For this review, take the finished solid that the model builds, in its own axes (mm). Face numbers are marked on the shaded views. Coordinates: 2 decimals unless noted, no trailing zeros. Loops run counter-clockwise (first coordinate to the right, second up) from the corner with the lowest first, then second, coordinate; pieces in that order, holes last. Notation, with made-up numbers: M 77.5,-0.5 L 113.5,-0.5 A18 ccw 113.5,14.5 Z; hole C 51.25,-20.5 d3. An arc over 180 degrees is marked long. Use one line per item in the form item = value.
Autodesk Inventor part; units mm, degrees
ref_plane "Work Plane1" through (9, 0, 0) normal (1, 0, 0) x (0, 0, -1)
ref_plane "YZ Plane" through (0, 0, 0) normal (1, 0, 0) x (0, 1, 0)
ref_plane "XZ Plane" through (0, 0, 0) normal (0, 1, 0) x (-1, 0, 0)
sketch "Sketch1" plane through (0, 0, 0) normal (1, 0, 0) x (0, 1, 0)
  line L0 (-15, 75) -> (15, 75)
  line L1 (15, 75) -> (15, -75)
  line L2 (15, -75) -> (-15, -75)
  line L3 (-15, -75) -> (-15, 75)
  line L4 (-15, 75) -> (15, -75) construction
  line L5 (15, 75) -> (-15, -75) construction
  line L6 (15, 64.89637) -> (15, 43.985813)
  line L7 (-15, 43.985813) -> (-15, 64.193072)
  line L8 (-21, 0) -> (21, 0)
  line L9 (0, -105) -> (0, 105)
  line L10 (-15, -62.009619) -> (-7.5, -49.019238)
  line L11 (-7.5, -49.019238) -> (7.5, -49.019238)
  line L12 (7.5, -49.019238) -> (15, -62.009619)
  line L13 (15, -62.009619) -> (7.5, -75)
  line L14 (7.5, -75) -> (-7.5, -75)
  line L15 (-7.5, -75) -> (-15, -62.009619)
  line L16 (15, 62.009619) -> (7.5, 75)
  line L17 (-7.5, 75) -> (-15, 62.009619)
  point P0 (0, 0)
  point P1 (0, -62.009619)
  point P2 (-7.5, -75)
  point P3 (7.5, -75)
  point P4 (15, -62.009619)
  point P5 (15, 62.009619)
  point P6 (7.5, 75)
  point P7 (-7.5, 75)
  point P8 (-15, 62.009619)
  dimension "d0" = 30
  dimension "d1" = 150
extrude "Extrusion1" add sketch "Sketch1" along normal blind 4 contours L0 L9 L8 L3 L17 | L0 L16 L1 L8 L9 | L9 L11 L10 L3 L8 | L8 L1 L12 L11 L9 | L11 L12 L13 L2 L9 | L9 L2 L15 L10 L11
sketch "Sketch2" plane through (4, 0, 0) normal (1, 0, 0) x (0, 0, -1)
  line L0 (62.009619, 15) -> (-62.009619, 15)
  line L1 (62.009619, 15) -> (-62.009619, 15)
  line L2 (-62.009619, -15) -> (62.009619, -15)
  line L3 (-105, 0) -> (105, 0)
  line L4 (0, -21) -> (0, 21)
  line L5 (-68.504809, 4.618802) -> (-64.504809, 2.309401)
  line L6 (-64.504809, 2.309401) -> (-64.504809, -2.309401)
  line L7 (-64.504809, -2.309401) -> (-68.504809, -4.618802)
  line L8 (-68.504809, -4.618802) -> (-72.504809, -2.309401)
  line L9 (-72.504809, -2.309401) -> (-72.504809, 2.309401)
  line L10 (-72.504809, 2.309401) -> (-68.504809, 4.618802)
  line L11 (68.504809, 4.618802) -> (64.504809, 2.309401)
  line L12 (64.504809, 2.309401) -> (64.504809, -2.309401)
  line L13 (64.504809, -2.309401) -> (68.504809, -4.618802)
  line L14 (68.504809, -4.618802) -> (72.504809, -2.309401)
  line L15 (72.504809, -2.309401) -> (72.504809, 2.309401)
  line L16 (72.504809, 2.309401) -> (68.504809, 4.618802)
  line L17 (-75, 7.5) -> (-75, -7.5)
  line L18 (-62.009619, -15) -> (62.009619, -15)
  line L19 (-62.009619, 15) -> (-62.009619, -15)
  line L20 (-75, 7.5) -> (-75, -7.5)
  line L21 (-75, 0) -> (-62.009619, 0)
  point P0 (0, 0)
  point P1 (68.504809, 0)
  point P2 (-68.504809, 0)
  dimension "d8" = 8
sketch "Sketch2 outline for Extrusion3" plane through (4, 0, 0) normal (1, 0, 0) x (0, 0, -1)
  line L0 (68.504809, -4.618802) -> (72.504809, -2.309401)
  line L1 (64.504809, -2.309401) -> (68.504809, -4.618802)
  line L2 (64.504809, 2.309401) -> (64.504809, -2.309401)
  line L3 (68.504809, 4.618802) -> (64.504809, 2.309401)
  line L4 (72.504809, 2.309401) -> (68.504809, 4.618802)
  line L5 (72.504809, -2.309401) -> (72.504809, 2.309401)
  line L6 (-64.504809, 2.309401) -> (-68.504809, 4.618802)
  line L7 (-64.504809, -2.309401) -> (-64.504809, 2.309401)
  line L8 (-68.504809, -4.618802) -> (-64.504809, -2.309401)
  line L9 (-72.504809, -2.309401) -> (-68.504809, -4.618802)
  line L10 (-72.504809, 2.309401) -> (-72.504809, -2.309401)
  line L11 (-68.504809, 4.618802) -> (-72.504809, 2.309401)
extrude "Extrusion3" add sketch "Sketch2 outline for Extrusion3" along normal blind 15
sketch "Sketch3" plane through (19, 0, 0) normal (1, 0, 0) x (0, 0, -1)
  line L0 (-64.504809, 2.309401) -> (-68.504809, 4.618802)
  line L1 (-68.504809, -4.618802) -> (-64.504809, -2.309401)
  line L2 (-64.504809, -2.309401) -> (-64.504809, 2.309401)
  line L3 (-64.504809, -2.309401) -> (-68.504809, -4.618802)
  circle A0 centre (-68.504809, 0) radius 1.55
  line L4 (0, -21) -> (0, 21)
  circle A1 centre (68.504809, 0) radius 1.55
  line L5 (-68.504809, 4.618802) -> (-68.504809, -4.618802)
  point P0 (0, 0)
  dimension "d12" = 3.1
extrude "Extrusion4" cut sketch "Sketch3" against normal through all contours L5 A0 | A0 L5 | A1
ref_plane "Work Plane1" through (9, 0, 0) normal (1, 0, 0) x (0, 0, -1)
sketch "Sketch4" plane through (9, 0, 0) normal (-1, 0, 0) x (0, 0, 1)
  circle A0 centre (-68.504809, 0) radius 1.55
  circle A1 centre (68.504809, 0) radius 1.55
  circle A2 centre (-68.504809, 0) radius 3.05
  circle A3 centre (68.504809, 0) radius 3.05
  point P0 (0, 0)
  dimension "d15" = 6.1
sketch "Sketch4 outline for Extrusion5" plane through (9, 0, 0) normal (-1, 0, 0) x (0, 0, 1)
  circle A0 centre (68.504809, 0) radius 3.05
  circle A1 centre (-68.504809, 0) radius 3.05
extrude "Extrusion5" cut sketch "Sketch4 outline for Extrusion5" against normal blind 2.2 draft -32.5
sketch "Sketch5" plane through (0, 0, 0) normal (-1, 0, 0) x (0, 0, 1)
  circle A0 centre (-68.504809, 0) radius 3.05
  circle A1 centre (68.504809, 0) radius 3.05
  point P0 (0, 0)
extrude "Extrusion6" cut sketch "Sketch5" against normal up to surface (9 mm away)
sketch "Sketch8" plane through (0, 0, 0) normal (-1, 0, 0) x (0, 0, 1)
  circle A0 centre (-35, 0) radius 2.1
  line L0 (-75, -7.5) -> (-75, 7.5)
  line L1 (0, -21) -> (0, 21)
  line L2 (75, 7.5) -> (75, -7.5)
  line L3 (-105, 0) -> (105, 0)
  point P0 (0, 0)
  dimension "d26" = 40
  dimension "d27" = 4.2
extrude "Extrusion7" cut sketch "Sketch8" against normal through all
equation "\"d0\" = BodyHeight"
equation "\"d1\" = BodyLength"
equation "\"d2\" = SideThickness"
equation "\"d8\" = M3ScrewInsertBrim"
equation "\"d9\" = WheeGuardlSlotWidth"
equation "\"d12\" = M3ScrewDia"
equation "\"d15\" = M3ScrewHeadDia"
equation "\"d16\" = M3ScrewHeadDepth"
equation "\"d17\" = M3ScrewHeadTaper"
equation "\"d26\" = DriveMotorOffset"
equation "\"d27\" = DriveMotorHoleDia"
properties part number "HexWheelGuard" material "H TPU"
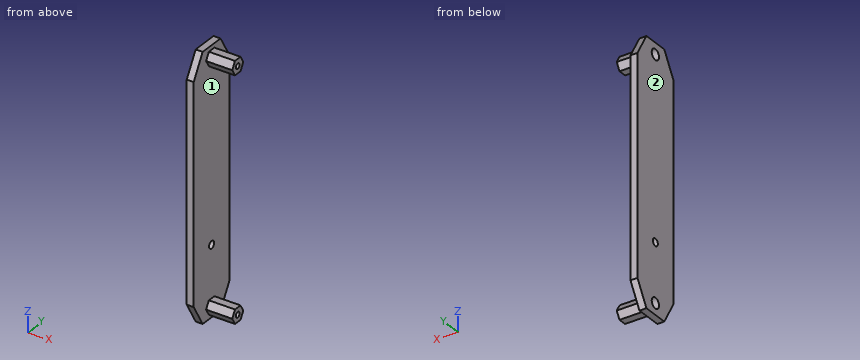
1. Consider section A-A on x = 13.5. Write out the cut boundary in (y, z), plus the area to 3 significant figures.
Computed values:
outline = M -4.62,-68.5 L -2.31,-72.5 L 2.31,-72.5 L 4.62,-68.5 L 2.31,-64.5 L -2.31,-64.5 Z; M -4.62,68.5 L -2.31,64.5 L 2.31,64.5 L 4.62,68.5 L 2.31,72.5 L -2.31,72.5 Z; hole C 0,-68.5 d3.1; hole C 0,68.5 d3.1
area = 95.8 mm2
2. For pin 1 Ø10 at (y, z) = (0, 68.5) entering from -X; pin 2 Ø2.5 at (x, y) = (8, 0.5) entering from -Z; pin 3 Ø3.5 at (x, y) = (12, 0.5) entering from +Z; pin 4 Ø3.5 at (y, z) = (0, -68.5) entering from -X, all flat-tipped, find the tip position at first contact; note any pin that passes through.
Computed values:
pin_1 = 0
pin_2 = -72.5
pin_3 = 72.5
pin_4 = 11.03
3. Wall thickness on line 1 along Z through (x, y) = (15.25, 2); line 2 along Z through (x, y) = (10.25, 2); line 3 along Y through (x, z) = (1.15, -35): over which ranges is each line inside the solid? List them lowest first. Write a range as from..to.
Computed values:
line_1 = -72.5..-64.5, 64.5..72.5
line_2 = -72.5..-69.54, -67.47..-64.5, 64.5..67.47, 69.54..72.5
line_3 = -15..-2.1, 2.1..15
4. Consider section C-C on y = 0. State how many separate pieces and enclosed holes the cut face has, plus the area to 3 significant figures.
Computed values:
separate_pieces = 4
enclosed_holes = 0
area = 644 mm2
5. Draft analysis for pull direction Z (two halves, no side actions). For the marked faces 1 and 2, state which applies: +Z half, -Z half, draft (parallel to the pull), parting line (faces both ways), or undercut.
Computed values:
face_1 = undercut
face_2 = draft
6. Consider section D-D on z = -16. Write out the cut boundary in (x, y), plus the area to 3 significant figures.
Computed values:
outline = M 0,-15 L 4,-15 L 4,15 L 0,15 Z
area = 120 mm2
7. Consider section B-B on z = -35. Write out the cut boundary in (x, y), plus the area to 3 significant figures.
Computed values:
outline = M 0,-15 L 4,-15 L 4,-2.1 L 0,-2.1 Z; M 0,2.1 L 4,2.1 L 4,15 L 0,15 Z
area = 103 mm2
